Can you work these out from the model? Positions are in its coordinate system, mm. Face numbers are marked on the shaded views. A direction names the side the tool comes from. Round coordinates to 2 decimals unless told otherwise and drop trailing zeros. Loops run counter-clockwise (first coordinate to the right, second up) from the corner with the lowest first, then second, coordinate; pieces in that order, holes last. Notation, with made-up numbers: (-38.5, 61) -> (-32.5, 61) arc R8 cw to (-32.5, 73) -> close; hole circle Ø11 at (36.25, 33.25). An arc over 180 degrees is marked (long way). Use a Markdown table: item, result.
from build123d import *

# Parameters (mm, degrees)
SKETCH2_W           = 23
SKETCH2_H           = 52.25
SKETCH2_W_2         = 20
SKETCH2_H_2         = 49.25
BOSS_EXTRUDE1_DEPTH = 7.5
SKETCH3_W           = 23
SKETCH3_H           = 52.25
BOSS_EXTRUDE2_DEPTH = 5
SKETCH4_W           = 6
SKETCH4_H           = 4.5
CUT_EXTRUDE1_DEPTH  = 1.5
CUT_EXTRUDE2_DEPTH  = 72.5
CUT_EXTRUDE3_START  = -3
CUT_EXTRUDE3_DEPTH  = 3
CUT_EXTRUDE4_DEPTH  = 3


# Read off the part's stored shape, not the designer's step: Cut-Extrude3
with BuildPart() as part:
    # Sketch2 → Boss-Extrude1 (new body)
    with BuildSketch(Plane(origin=(0, 0, 0), x_dir=(1, 0, 0), z_dir=(0, 1, 0))):
        with Locations((10, 25.375)):
            Rectangle(SKETCH2_W, SKETCH2_H)
        with Locations((10, 25.375)):
            Rectangle(SKETCH2_W_2, SKETCH2_H_2, mode=Mode.SUBTRACT)
    extrude(amount=BOSS_EXTRUDE1_DEPTH)

    # Sketch3 → Boss-Extrude2 (add)
    with BuildSketch(Plane.XZ):
        with Locations((10, -25.375)):
            Rectangle(SKETCH3_W, SKETCH3_H)
    extrude(amount=BOSS_EXTRUDE2_DEPTH)

    # Sketch4 → Cut-Extrude1 (cut)
    with BuildSketch(Plane(origin=(0, 0, -0.75), x_dir=(-1, 0, 0), z_dir=(0, 0, -1))):
        with Locations((-10, 2.25)):
            Rectangle(SKETCH4_W, SKETCH4_H)
    extrude(amount=-CUT_EXTRUDE1_DEPTH, mode=Mode.SUBTRACT)

    # Sketch5 → Cut-Extrude2 (cut)
    with BuildSketch(Plane(origin=(0, 0, -51.5), x_dir=(-1, 0, 0), z_dir=(0, 0, -1))):
        with BuildLine():
            Line((1.5, -5), (-21.5, -5))
            add(Edge.make_bspline(
                [(1.5, -5), (-10, -2), (-21.5, -5)],
                knots=[0, 0, 0, 1, 1, 1], degree=2))
        make_face()
    extrude(amount=-CUT_EXTRUDE2_DEPTH, mode=Mode.SUBTRACT)

    # Cut-Extrude3 outline → Cut-Extrude3 (cut)
    with BuildSketch(Plane(origin=(0, 0, -41.5), x_dir=(-1, 0, 0), z_dir=(0, 0, -1)).offset(CUT_EXTRUDE3_START)):
        with BuildLine():
            add(Edge.make_bspline(
                [(1.500000004, -4.225305609), (0.595466246, -3.993211731), (-1.297330219, -3.56483897), (-5.125081209, -2.941229912), (-10, -2.622513392), (-14.874918791, -2.941229912), (-18.702669782, -3.56483897), (-20.595466246, -3.993211731), (-21.500000004, -4.225305609)],
                knots=[0.499397619, 0.499397619, 0.499397619, 0.499397619, 0.499540721, 0.499693814, 0.5, 0.500306186, 0.500459279, 0.500602381, 0.500602381, 0.500602381, 0.500602381], degree=3))
            Line((1.500000004, -4.225305609), (1.5, -2.420629216))
            add(Edge.make_bspline(
                [(1.5, -2.420629216), (0.70515637, -2.224171116), (-1.108540102, -1.822242739), (-4.935012294, -1.198704697), (-10, -0.867469997), (-15.064987706, -1.198704697), (-18.891459898, -1.822242739), (-20.70515637, -2.224171116), (-21.499999999, -2.420629215)],
                knots=[0.499419719, 0.499419719, 0.499419719, 0.499419719, 0.499540721, 0.499693814, 0.5, 0.500306186, 0.500459279, 0.500580281, 0.500580281, 0.500580281, 0.500580281], degree=3))
            Line((-21.499999999, -2.420629215), (-21.500000004, -4.225305609))
        make_face()
    extrude(amount=CUT_EXTRUDE3_DEPTH, mode=Mode.SUBTRACT)

    # Sketch7 → Cut-Extrude4 (cut)
    with BuildSketch(Plane.XY.offset(-9.25)):
        with BuildLine():
            Line((-1.499999999, -2.420629215), (-1.500000004, -4.225305609))
            add(Edge.make_bspline(
                [(-1.500000004, -4.225305609), (-0.595466246, -3.993211731), (1.297330219, -3.56483897), (5.125081209, -2.941229912), (10, -2.622513392), (14.874918791, -2.941229912), (18.702669782, -3.56483897), (20.595466246, -3.993211731), (21.500000004, -4.225305609)],
                knots=[0.499397619, 0.499397619, 0.499397619, 0.499397619, 0.499540721, 0.499693814, 0.5, 0.500306186, 0.500459279, 0.500602381, 0.500602381, 0.500602381, 0.500602381], degree=3))
            Line((21.500000004, -4.225305609), (21.499999999, -2.420629215))
            add(Edge.make_bspline(
                [(21.499999999, -2.420629215), (20.70515637, -2.224171116), (18.891459898, -1.822242739), (15.064987706, -1.198704697), (10, -0.867469997), (4.935012294, -1.198704697), (1.108540102, -1.822242739), (-0.70515637, -2.224171116), (-1.499999999, -2.420629215)],
                knots=[0.499419719, 0.499419719, 0.499419719, 0.499419719, 0.499540721, 0.499693814, 0.5, 0.500306186, 0.500459279, 0.500580281, 0.500580281, 0.500580281, 0.500580281], degree=3))
        make_face()
    extrude(amount=-CUT_EXTRUDE4_DEPTH, mode=Mode.SUBTRACT)


solid = part.part
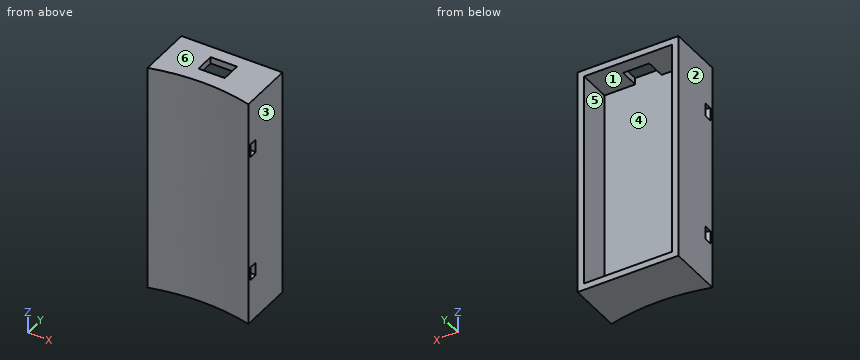
1. I want a section at A-A (y = 6). Please give me the cut outline in (x, z).
Answer sheet:
| item | result |
|---|---|
| outline | (-1.5, -51.5) -> (21.5, -51.5) -> (21.5, 0.75) -> (-1.5, 0.75) -> close; hole (0, -50) -> (20, -50) -> (20, -0.75) -> (0, -0.75) -> close |
2. I need wall thicknesses on line 1 (Z direction, x = 13.5, y = -2.25); line 2 (X direction, y = 5.5, z = -44); line 3 (Y direction, x = 10.5, z = -39). Which ranges of each line are inside material? Lowest first, please.
Answer sheet:
| item | result |
|---|---|
| line 1 | z = -51.5 to -41.5, -38.5 to -12.25, -9.25 to 0.75 |
| line 2 | x = -1.5 to 0, 20 to 21.5 |
| line 3 | y = -3.5 to -2.75, -1 to 0 |
3. I want a section at C-C (x = 8). State how many separate pieces and enclosed holes the cut face has, plus the area to 3 significant figures.
Answer sheet:
| item | result |
|---|---|
| separate pieces | 2 |
| enclosed holes | 2 |
| area | 190 mm² |
4. I want a section at B-B (y = 2.75). Please give me the cut outline in (x, z).
Answer sheet:
| item | result |
|---|---|
| outline | (-1.5, -51.5) -> (21.5, -51.5) -> (21.5, 0.75) -> (13, 0.75) -> (13, -0.75) -> (20, -0.75) -> (20, -50) -> (0, -50) -> (0, -0.75) -> (7, -0.75) -> (7, 0.75) -> (-1.5, 0.75) -> close |
5. Will these pins go through, and if not, where does the flat tip stop? pin 1 Ø0.8 at (x, z) = (9.5, 0) entering from -Y; pin 2 Ø1 at (x, z) = (18, -20.5) entering from -Y.
Answer sheet:
| item | result |
|---|---|
| pin 1 | stops at y = -3.51 |
| pin 2 | stops at y = -4.32 |
6. Which directions (+Z, -Z, +X, -X, +Y, -Y) give clear straight access to the entire face, cutting with the end or side of a thin tool? Please do the marked faces 1 and 2.
Answer sheet:
| item | result |
|---|---|
| face 1 | +Y |
| face 2 | +Z, -Z, -X, +Y, -Y |
7. If we mould it in two halves opening along Z, with no side actions, what happens to the marked faces 3, 4, 5 and 6? For each: +Z half, -Z half, draft (parallel to the pull), parting line (faces both ways), or undercut.
Answer sheet:
| item | result |
|---|---|
| face 3 | draft |
| face 4 | undercut |
| face 5 | undercut |
| face 6 | +Z half |
